Verification items for the finished model (mm, model axes). A direction names the side the tool comes from. Round coordinates to 2 decimals unless told otherwise and drop trailing zeros. Write each loop counter-clockwise with the first axis right and the second up, starting at its lowest first coordinate (ties: lowest second). Pieces come first, ordered by that corner, then holes. Notation, with made-up numbers: M 39.5,73.25 L 70.5,73.25 A14 cw 70.5,94.25 Z; hole C 83.5,-1 d4. An arc over 180 degrees is marked long. Answer in a Markdown table with one row per item. Add a question column.
1. Draft check along Z on faces 1 (the cylindrical face through (13.089, 5.07, 57.532)), 2 (the flat face through (-1, 5, 100)), 3 (the flat face through (-1, 10, 65)), 4 (the flat face through (-55, 15, -60)). Enter one of: pulls with the +Z half, pulls with the -Z half, needs draft (parallel to the pull), parting line crosses it, or undercut.
2. Sectioned sample at B-B on z = 75. Record the cut outline in (x, y), plus the area to 3 significant figures.
3. Material ranges on probe 1 along X at (y, z) = (19.25, -81); probe 2 along Z at (x, y) = (51.75, 4.75); probe 3 along Z at (x, y) = (9.5, 3.25), recorded low to high.
4. Go/stop test with flat-tipped pins: pin 1 Ø9 at (x, z) = (-54, -83) entering from +Y; pin 2 Ø2 at (x, y) = (-22, 12.5) entering from +Z; pin 3 Ø1 at (x, y) = (48, 17.5) entering from -Z. Record where each tip stops, or that it passes through.
5. Sectioned sample at C-C on x = -73. Record the cut outline in (y, z).
6. Sectioned sample at A-A on x = -46. Record the cut outline in (y, z).
7. Set-up check for faces 5 (the flat face through (34.976, 15, 46)), 6 (the flat face through (-68, 15, 80.062)), 7 (the flat face through (40, 15, -80)): record each of +Z, -Z, +X, -X, +Y, -Y from which the full face is reachable in a straight line by a thin tool's end or side.
Autodesk Inventor part; units mm, degrees
ref_plane "YZ Plane" through (0, 0, 0) normal (1, 0, 0) x (0, 1, 0)
ref_plane "XZ Plane" through (0, 0, 0) normal (0, 1, 0) x (-1, 0, 0)
ref_plane "XY Plane" through (0, 0, 0) normal (0, 0, 1) x (1, 0, 0)
sketch "Boceto1" plane through (0, 0, 0) normal (0, 1, 0) x (-1, 0, 0)
  line L0 (100, 100) -> (-100, 100)
  line L1 (-100, 100) -> (-100, -100)
  line L2 (-100, -100) -> (100, -100)
  line L3 (100, -100) -> (100, 100)
  line L4 (100, 100) -> (-100, -100) construction
  line L5 (-100, 100) -> (100, -100) construction
  point P0 (0, 0)
  dimension "d0" = 200
  dimension "d1" = 200
extrude "Extrusión1" add sketch "Boceto1" along normal blind 20
sketch "Boceto2" plane through (0, 20, 0) normal (0, 1, 0) x (1, 0, 0)
  circle A0 centre (-11.5239, -30.0616) radius 3
  circle A1 centre (11.4761, -30.0616) radius 3
  circle A2 centre (-11.5239, -60.0616) radius 3
  circle A3 centre (11.4761, -60.0616) radius 3
  line L0 (-0.0239, -45.0616) -> (-35.0239, -45.0616)
  line L1 (-35.0239, -45.0616) -> (-35.0239, -80.0616)
  line L2 (-0.0239, -45.0616) -> (34.9761, -45.0616)
  line L3 (-11.5239, -30.0616) -> (11.4761, -60.0616)
  line L4 (-11.5239, -60.0616) -> (11.4761, -30.0616)
  line L5 (34.9761, -11.0616) -> (-35.0239, -11.0616)
  line L6 (-35.0239, -11.0616) -> (-35.0239, -80.0616)
  line L7 (34.9761, -80.0616) -> (34.9761, -11.0616)
  line L8 (-105, -100.0616) -> (105, -100.0616)
  line L9 (-105.0239, -80.0616) -> (104.9761, -80.0616)
  line L10 (-35.0239, -80.0616) -> (34.9761, -80.0616)
  line L11 (105, -100.0616) -> (95.8154, -100.0616)
  line L12 (-105.0239, -80.0616) -> (104.9761, -80.0616)
  line L13 (105, -80.0616) -> (-105, -80.0616)
  line L14 (-105, -100.0616) -> (105, -100.0616)
  line L15 (105, -90.0616) -> (94.0798, -90.0616)
  line L16 (-105, -100.0616) -> (105, -100.0616)
  line L17 (-105, -80.0616) -> (105, -80.0616)
  line L18 (105, -80.0616) -> (105, -100.0616)
  line L19 (105, -100.0616) -> (-105, -100.0616)
  line L20 (-105, -100.0616) -> (-105, -80.0616)
  line L21 (-100, 100) -> (-100, -100)
  line L22 (-100, -100) -> (100.4077, -100)
  point P0 (0, 0)
  point P1 (0, -10.0616)
  point P2 (0, -90.0616)
  point P3 (-0.0478, -80.0616)
  dimension "d4" = 20
  dimension "d5" = 20
  dimension "d6" = 30
  dimension "d7" = 30
  dimension "d8" = 20
  dimension "d9" = 35
  dimension "d10" = 35
  dimension "d11" = 69
extrude "Extrusión2" cut sketch "Boceto2" against normal blind 10
sketch "Boceto3" plane through (0, 20, 0) normal (0, 1, 0) x (1, 0, 0)
  circle A0 centre (-11.5239, -30.0616) radius 3
  circle A1 centre (-11.5239, -30.0616) radius 3
  circle A2 centre (11.4761, -30.0616) radius 3
  circle A3 centre (11.4761, -30.0616) radius 3
  circle A4 centre (11.4761, -60.0616) radius 3
  circle A5 centre (11.4761, -60.0616) radius 3
  circle A6 centre (-11.5239, -60.0616) radius 3
  point P0 (0, 0)
extrude "Extrusión3" cut sketch "Boceto3" against normal blind 20
sketch "Boceto4" plane through (0, 20, 0) normal (0, 1, 0) x (1, 0, 0)
  circle A0 centre (-51.75, 78.25) radius 1.75
  line L0 (-50, 70) -> (-60, 70)
  line L1 (-60, 70) -> (-60, 80)
  line L2 (-60, 80) -> (-50, 80)
  line L3 (-50, 80) -> (-50, 70)
  line L4 (-50, 70) -> (-60, 80) construction
  line L5 (-60, 70) -> (-50, 80) construction
  line L6 (-105, 90) -> (-105, -90)
  circle A1 centre (-58.25, 71.75) radius 1.75
  line L7 (0, 90) -> (0, 77.3124)
  circle A2 centre (51.75, 78.25) radius 1.75
  line L8 (50, 70) -> (60, 70)
  line L9 (60, 70) -> (60, 80)
  line L10 (60, 80) -> (50, 80)
  line L11 (50, 80) -> (50, 70)
  line L12 (50, 70) -> (60, 80) construction
  line L13 (60, 70) -> (50, 80) construction
  circle A3 centre (58.25, 71.75) radius 1.75
  line L14 (100, 100) -> (-100, 100)
  line L15 (-100, 100) -> (-100, -80.0616)
  line L16 (100, -80.0616) -> (100, 100)
  point P0 (0, 0)
  point P1 (0, 0)
  point P2 (-60, 75)
  point P3 (60, 75)
  dimension "d16" = 3.5
  dimension "d18" = 1.75
  dimension "d19" = 1.75
  dimension "d20" = 1.75
  dimension "d21" = 1.75
  dimension "d22" = 10
  dimension "d23" = 10
  dimension "d25" = 20
  dimension "d26" = 40
  dimension "d27" = 40
hole "Agujero1" at (-58.25, 20, -71.75) at (-51.75, 20, -78.25) at (58.25, 20, -71.75) at (51.75, 20, -78.25) direction (0, -1, 0) diameter 3.5 end through all
sketch "Boceto5" plane through (0, 20, 0) normal (0, 1, 0) x (1, 0, 0)
  line L0 (0, 90) -> (0, 68.25)
  circle A0 centre (-51.75, 78.25) radius 1.75
  line L1 (-50, 78.25) -> (-50, 100)
  circle A1 centre (-58.25, 71.75) radius 1.75
  line L2 (-60, 71.75) -> (-60, 100)
  line L3 (-60, 100) -> (-70, 100)
  line L4 (-50, 100) -> (-40, 100)
  line L5 (-40, 100) -> (-40, 60)
  line L6 (-40, 60) -> (-70, 60)
  line L7 (-70, 60) -> (-70, 100)
  line L8 (-70, 100) -> (-40, 100)
  circle A2 centre (51.75, 78.25) radius 1.75
  line L9 (50, 78.25) -> (50, 100)
  circle A3 centre (58.25, 71.75) radius 1.75
  line L10 (60, 71.75) -> (60, 100)
  line L11 (60, 100) -> (70, 100)
  line L12 (50, 100) -> (40, 100)
  line L13 (40, 100) -> (40, 60)
  line L14 (40, 60) -> (70, 60)
  line L15 (70, 60) -> (70, 100)
  line L16 (70, 100) -> (40, 100)
  point P0 (0, 0)
  dimension "d38" = 10
  dimension "d39" = 10
  dimension "d40" = 40
extrude "Extrusión4" cut sketch "Boceto5" against normal blind 10
properties part number "base_front_red"
Geometry check:
| question | item | result |
|---|---|---|
| 1 | face 1 | undercut |
| 1 | face 2 | pulls with the +Z half |
| 1 | face 3 | needs draft |
| 1 | face 4 | pulls with the -Z half |
| 2 | outline | M -100,0 L 100,0 L 100,20 L 34.98,20 L 34.98,10 L -35.02,10 L -35.02,20 L -100,20 Z |
| 2 | area | 3,300 mm2 |
| 3 | probe 1 | x = -100 to -70, -40 to 40, 70 to 100 |
| 3 | probe 2 | z = -100 to -80, -76.5 to 100 |
| 3 | probe 3 | z = -100 to 27.8, 32.32 to 57.8, 62.32 to 100 |
| 4 | pin 1 | stops at y = 10 |
| 4 | pin 2 | stops at z = 11.06 |
| 4 | pin 3 | stops at z = -60 |
| 5 | outline | M 0,-100 L 20,-100 L 20,80.06 L 10,80.06 L 10,100 L 0,100 Z |
| 6 | outline | M 0,-100 L 10,-100 L 10,-60 L 20,-60 L 20,80.06 L 10,80.06 L 10,100 L 0,100 Z |
| 7 | face 5 | +Z, +Y |
| 7 | face 6 | +Z, +X, -X, +Y |
| 7 | face 7 | -Z, +Y |
